```python
from build123d import *

# Parameters (mm, degrees)
CUT_HEX_START     = 3.175
SKETCH2_OUTSIDE_W = 35.848
SKETCH2_OUTSIDE_H = 35.848
CUT_HEX_DEPTH     = 26.4


with BuildPart() as part:
    # Sketch1 → Revolve1 (revolve)
    with BuildSketch(Plane(origin=(0, 0, 0), x_dir=(0, 0, -1), z_dir=(1, 0, 0)), mode=Mode.PRIVATE) as revolve1_sk:
        Polygon((-20.744473185, 12.7), (0, 12.7), (0, 6.35), (-22.225, 6.35), (-22.225, 9.525), align=None)
    revolve(revolve1_sk.sketch.rotate(Axis((0, 0, 34.597150245), (0, 0, -1)), 90), axis=Axis((0, 0, 34.597150245), (0, 0, -1)))

    # Sketch2 outside → Cut-HEX (cut, through all)
    with BuildSketch(Plane.XY.offset(CUT_HEX_START)):
        Rectangle(SKETCH2_OUTSIDE_W, SKETCH2_OUTSIDE_H)
        Polygon((9.525, -5.499261314), (9.525, 5.499261314), (0, 10.998522628), (-9.525, 5.499261314), (-9.525, -5.499261314), (0, -10.998522628), align=None, mode=Mode.SUBTRACT)
    extrude(amount=CUT_HEX_DEPTH, mode=Mode.SUBTRACT)


solid = part.part
```
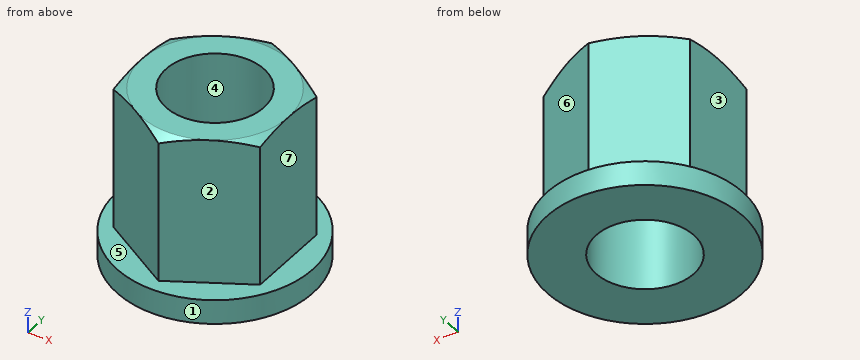
Check sheet for the modelled part. Datum: model origin and axes. Units: mm. Face numbers are marked on the shaded views. A direction names the side the tool comes from. Round coordinates to 2 decimals unless told otherwise and drop trailing zeros. Write each loop counter-clockwise with the first axis right and the second up, starting at its lowest first coordinate (ties: lowest second). Pieces come first, ordered by that corner, then holes. Notation, with made-up numbers: (44, 61.5) -> (82, 61.5) arc R12 ccw to (82, 79.5) -> close; hole circle Ø2 at (-3.75, 11.5). An arc over 180 degrees is marked (long way). Put each result on its own line as item: value.
(1) Material ranges on line 1 (X direction, y = 3.25, z = 11.25) (3 decimals); line 2 (Z direction, x = 1.5, y = 10.5) (3 decimals); line 3 (Y direction, x = 2, z = 18.75), recorded low to high.
Values found:
line 1: x = -9.525 to -5.455, 5.455 to 9.525
line 2: z = 0 to 3.175
line 3: y = -9.84 to -6.03, 6.03 to 9.84
(2) Go/stop test with flat-tipped pins: pin 1 Ø10 at (x, y) = (0, 0) entering from -Z; pin 2 Ø3 at (x, z) = (5.5, 17) entering from +Y; pin 3 Ø12 at (y, z) = (-1.5, 16) entering from +X (3 decimals); pin 4 Ø5 at (y, z) = (3.5, 19) entering from -X (3 decimals). Record where each tip stops, or that it passes through.
Values found:
pin 1: passes through
pin 2: stops at y = 8.69
pin 3: stops at x = 9.525
pin 4: stops at x = -9.525
(3) Tool access check on the marked faces 5, 6 and 7. Record the directions out of +Z, -Z, +X, -X, +Y, -Y that give a thin tool (end or side, any length) a straight path to the whole face; none if there is none.
Values found:
face 5: +Z
face 6: +Z, +X, +Y
face 7: +Z, +X, +Y, -Y
(4) Mould release check, pull along Y, two halves, no side actions. Record for the marked faces 1, 2, 3 and 4: released by +Y, released by -Y, zero draft, split by the parting line, or undercut.
Values found:
face 1: split by the parting line
face 2: released by -Y
face 3: zero draft
face 4: undercut
(5) Sectioned sample at A-A (z = 17.5). Enter the section's corners in (x, y) (3 decimals), plus the area to 3 significant figures.
Values found:
outline: (-9.525, -5.499) -> (0, -10.999) -> (9.525, -5.499) -> (9.525, 5.499) -> (0, 10.999) -> (-9.525, 5.499) -> close; hole circle Ø12.7 at (0, 0)
area: 188 mm^2
